```python
from build123d import *

# Parameters (mm, degrees)
SKETCH1_W           = 45
SKETCH1_H           = 4
BOSS_EXTRUDE1_DEPTH = 18
SKETCH2_R           = 8.5
CUT_EXTRUDE2_DEPTH  = 0.5
SKETCH3_R           = 3
CUT_EXTRUDE3_DEPTH  = 4.5
SKETCH4_R           = 2.5
CUT_EXTRUDE4_DEPTH  = 5
SKETCH6_R           = 0.8
CUT_EXTRUDE6_DEPTH  = 4.5
FILLET1_R           = 10
SKETCH7_R           = 5.2
CUT_EXTRUDE7_DEPTH  = 1.555


with BuildPart() as part:
    # Sketch1 → Boss-Extrude1 (new body)
    with BuildSketch(Plane(origin=(0, 0, 0), x_dir=(1, 0, 0), z_dir=(0, 1, 0))):
        with Locations((-22.5, 2)):
            Rectangle(SKETCH1_W, SKETCH1_H)
    extrude(amount=BOSS_EXTRUDE1_DEPTH)

    # Sketch2 → Cut-Extrude2 (cut)
    with BuildSketch(Plane.XY):
        with Locations((-22.5, 9)):
            Circle(SKETCH2_R)
    extrude(amount=-CUT_EXTRUDE2_DEPTH, mode=Mode.SUBTRACT)

    # Sketch3 → Cut-Extrude3 (cut, through all)
    with BuildSketch(Plane.XY.offset(-0.5)):
        with Locations((-22.5, 9)):
            Circle(SKETCH3_R)
    extrude(amount=-CUT_EXTRUDE3_DEPTH, mode=Mode.SUBTRACT)

    # Sketch4 → Cut-Extrude4 (cut, through all)
    with BuildSketch(Plane.XY):
        with Locations((-35.5, 9)):
            Circle(SKETCH4_R)
        with Locations((-9.5, 9)):
            Circle(SKETCH4_R)
    extrude(amount=-CUT_EXTRUDE4_DEPTH, mode=Mode.SUBTRACT)

    # Sketch6 → Cut-Extrude6 (cut, through all)
    with BuildSketch(Plane.XY.offset(-0.5)):
        with Locations((-22.5, 14)):
            Circle(SKETCH6_R)
        with Locations((-18.169872981, 11.5)):
            Circle(SKETCH6_R)
        with Locations((-18.169872981, 6.5)):
            Circle(SKETCH6_R)
        with Locations((-22.5, 4)):
            Circle(SKETCH6_R)
        with Locations((-26.830127019, 6.5)):
            Circle(SKETCH6_R)
        with Locations((-26.830127019, 11.5)):
            Circle(SKETCH6_R)
    extrude(amount=-CUT_EXTRUDE6_DEPTH, mode=Mode.SUBTRACT)

    # Fillet1
    fillet1_edges = [part.edges().sort_by_distance(p)[0] for p in [
        (-45, 18, -2),
        (0, 18, -2),
    ]]
    fillet(fillet1_edges, radius=FILLET1_R)

    # Sketch7 → Cut-Extrude7 (cut)
    with BuildSketch(Plane.XY):
        with Locations((-35.5, 9)):
            Circle(SKETCH7_R)
        with Locations((-9.5, 9)):
            Circle(SKETCH7_R)
    extrude(amount=-CUT_EXTRUDE7_DEPTH, mode=Mode.SUBTRACT)


solid = part.part
```
Verification items for the finished model (mm, model axes). A direction names the side the tool comes from. Give positions to 0.01 mm unless a question says otherwise; leave off trailing zeros. Order: outer loops, then holes, each group sorted by start corner. A loop starts at its lowest first (then second) coordinate and runs counter-clockwise, first axis right, second up. Notation, with made-up numbers: (61.5, 48) -> (88.5, 48) arc R22 ccw to (88.5, 65) -> close; hole circle Ø2 at (47.25, 24.25). An arc over 180 degrees is marked (long way). Use a Markdown table: item, result.
1) Depth check by flat-ended pin: pin 1 Ø8.5 at (x, y) = (-9.5, 9) entering from -Z; pin 2 Ø5 at (x, y) = (-23, 10) entering from +Z; pin 3 Ø3 at (x, y) = (-9, 10.5) entering from +Z (3 decimals); pin 4 Ø1.5 at (y, z) = (9, -3) entering from +X. Enter the tip coordinate at first touch or a pass-through.
Results:
| item | result |
|---|---|
| pin 1 | z = -4 |
| pin 2 | z = -0.5 |
| pin 3 | z = -1.555 |
| pin 4 | x = 0 |
2) Section check B-B, the plane x = -8. Record the boundary of the cut face in (y, z) (3 decimals), then the cut area to 3 significant figures.
Results:
| item | result |
|---|---|
| outline | (0, -4) -> (7, -4) -> (7, -1.555) -> (4.021, -1.555) -> (4.021, 0) -> (0, 0) -> close; (11, -4) -> (17.798, -4) -> (17.798, 0) -> (13.979, 0) -> (13.979, -1.555) -> (11, -1.555) -> close |
| area | 45.9 mm² |
3) Section check D-D, the plane x = -35.5. Record the boundary of the cut face in (y, z) (1 decimal).
Results:
| item | result |
|---|---|
| outline | (0, -4) -> (6.5, -4) -> (6.5, -1.6) -> (3.8, -1.6) -> (3.8, 0) -> (0, 0) -> close; (11.5, -4) -> (18, -4) -> (18, 0) -> (14.2, 0) -> (14.2, -1.6) -> (11.5, -1.6) -> close |
4) Section check C-C, the plane y = 1.75. Record the boundary of the cut face in (x, z).
Results:
| item | result |
|---|---|
| outline | (-45, -4) -> (0, -4) -> (0, 0) -> (-18.06, 0) -> (-18.06, -0.5) -> (-26.94, -0.5) -> (-26.94, 0) -> (-45, 0) -> close |
5) Tool access check on faces 1 (the cylindrical face through (-25.5, 9.1, -2.2)), 2 (the flat face through (-33, 10, -1.555)). Record the directions out of +Z, -Z, +X, -X, +Y, -Y that give a thin tool (end or side, any length) a straight path to the whole face; none if there is none.
Results:
| item | result |
|---|---|
| face 1 | +Z, -Z |
| face 2 | +Z |
6) Section check A-A, the plane z = -3.25. Give the number of separate pieces and of enclosed holes in the cut face, then the cut area to 3 significant figures.
Results:
| item | result |
|---|---|
| separate pieces | 1 |
| enclosed holes | 9 |
| area | 687 mm² |
7) Material ranges on probe 1 along Y at (x, z) = (-22.5, -2.2); probe 2 along X at (y, z) = (13.25, -0.3); probe 3 along X at (y, z) = (13.75, -1.45), recorded low to high.
Results:
| item | result |
|---|---|
| probe 1 | 0 to 3.2, 4.8 to 6, 12 to 13.2, 14.8 to 18 |
| probe 2 | -43.51 to -38.5, -32.5 to -29.86, -15.14 to -12.5, -6.5 to -1.49 |
| probe 3 | -43.18 to -37.62, -33.38 to -23.26, -21.74 to -11.62, -7.38 to -1.82 |
